```python
from build123d import *

# Parameters (mm, degrees)
F0_W      = 670
F0_H      = 678
F1_DEPTH  = 540
F2_R      = 31.5
F3_DEPTH  = 125
F4_W      = 290
F4_H      = 33
F5_DEPTH  = 670
F6_R      = 190
F7_DEPTH  = 670
F8_W      = 105.455173281
F8_H      = 190
F9_DEPTH  = 670
F11_DEPTH = 15


with BuildPart() as f1:
    # F0 (on Front) → F1 (new body)
    with BuildSketch(Plane.XZ):
        with Locations((1.9415970892, 64.8658148712)):
            Rectangle(F0_W, F0_H)
    extrude(amount=-F1_DEPTH)

    # F2 (on face) → F3 (cut)
    with BuildSketch(Plane.XY.offset(403.8658148712)):
        with Locations((1.9415970892, 457)):
            Circle(F2_R)
    extrude(amount=-F3_DEPTH, mode=Mode.SUBTRACT)

    # F4 (on face) → F5 (cut)
    with BuildSketch(Plane.YZ.offset(336.9415970892)):
        with Locations((395, 262.3658148712)):
            Rectangle(F4_W, F4_H)
    extrude(amount=-F5_DEPTH, mode=Mode.SUBTRACT)

    # F6 (on face) → F7 (cut)
    with BuildSketch(Plane.YZ.offset(336.9415970892)):
        with Locations((270, -4.1341851288)):
            Circle(F6_R)
    extrude(amount=-F7_DEPTH, mode=Mode.SUBTRACT)

    # F8 (on face) → F9 (cut)
    with BuildSketch(Plane.YZ.offset(336.9415970892)):
        with Locations((487.2724133595, -4.1341851288)):
            Rectangle(F8_W, F8_H)
    extrude(amount=-F9_DEPTH, mode=Mode.SUBTRACT)

    # F10 (on face) → F11 (cut)
    with BuildSketch(Plane.XZ):
        Polygon((-285.0584029108, 403.8658148712), (-333.0584029108, 403.8658148712), (-333.0584029108, 355.8658148712), (-45.7536410061, 64.8658148712), (-333.0584029108, -226.1341851288), (-333.0584029108, -274.1341851288), (-285.0584029108, -274.1341851288), (1.9415970892, 16.5571331991), (288.9415970892, -274.1341851288), (336.9415970892, -274.1341851288), (336.9415970892, -226.1341851288), (49.6368351844, 64.8658148712), (336.9415970892, 355.8658148712), (336.9415970892, 403.8658148712), (288.9415970892, 403.8658148712), (1.9415970892, 113.1744965432), align=None)
    extrude(amount=-F11_DEPTH, mode=Mode.SUBTRACT)


solid = f1.part
```
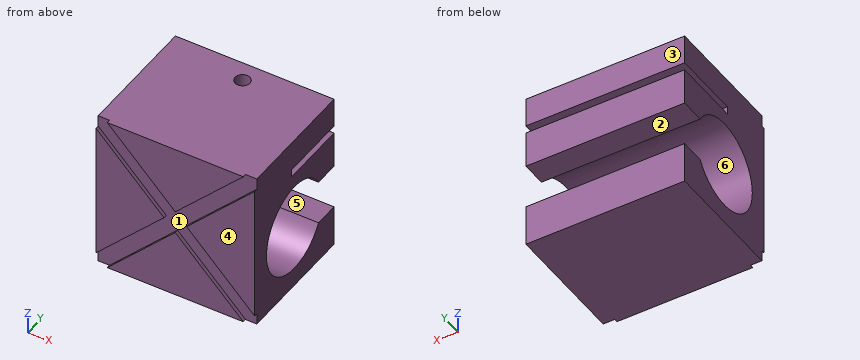
Could you check a few things on this model? Use its own coordinates, in mm. Face numbers are marked on the shaded views. A direction names the side the tool comes from. Round coordinates to 2 decimals unless told otherwise and drop trailing zeros. Order: outer loops, then holes, each group sorted by start corner. A loop starts at its lowest first (then second) coordinate and runs counter-clockwise, first axis right, second up. Notation, with made-up numbers: M -38.5,-10.5 L -20.5,-10.5 A7 cw -20.5,-1.5 Z; hole C 43,-8.5 d6. An arc over 180 degrees is marked long. One line per question, with ' | ' between items. Start each with the question number.
(1) Please list where these lines run through material, in increasing order: line 1 along Z through (x, y) = (99.5, 439); line 2 along Z through (x, y) = (-120, 270); line 3 along Y through (x, z) = (143.5, -67).
(2) Suppose I cut it at B-B on y = 123.5. List the corners of the cut face in (x, z) for me.
(3) Suppose I cut it at A-A on y = 498. List the corners of the cut face in (x, z) for me, then the cut area to 3 significant figures.
(4) Suppose I cut it at C-C on x = -20. List the corners of the cut face in (y, z) for me, then the cut area to 3 significant figures.
(5) Suppose I cut it at D-D on z = 316. List the corners of the cut face in (x, y) for me.
(6) For the marked faces 1, 2 and 3, which set-ups out of +Z, -Z, +X, -X, +Y, -Y let a thin tool reach every point of the face, with its end or its side?
(7) For P1, Ø2, axis at x = 55, z = 38, coming from the -Y side; P2, Ø16.5, axis at x = -14.5, z = 258.5, coming from the +Y side, each with a flat end and sliding along its axis, tell me the tip position at first contact or that it passes through.
(8) Thinking about a two-plate mould opening in Y: for the marked faces 4, 5 and 6, which applies, +Y half, -Y half, draft (parallel to the pull), parting line (faces both ways), or undercut?
Geometry results:
1) line 1: -274.13 to -99.13, 90.87 to 245.87, 278.87 to 403.87 | line 2: -274.13 to -194.13, 185.87 to 245.87, 278.87 to 403.87 | line 3: 15 to 90.7
2) outline: M -333.06,-274.13 L 336.94,-274.13 L 336.94,-125.12 L -333.06,-125.12 Z; M -333.06,116.85 L 336.94,116.85 L 336.94,403.87 L -333.06,403.87 Z
3) outline: M -333.06,-274.13 L 336.94,-274.13 L 336.94,-99.13 L -333.06,-99.13 Z; M -333.06,90.87 L 336.94,90.87 L 336.94,245.87 L -333.06,245.87 Z; M -333.06,278.87 L 336.94,278.87 L 336.94,403.87 L -333.06,403.87 Z | area: 305,000 mm²
4) outline: M 0,-274.13 L 540,-274.13 L 540,-99.13 L 434.54,-99.13 A190 cw long 434.54,90.87 L 540,90.87 L 540,245.87 L 250,245.87 L 250,278.87 L 434.4,278.87 L 434.4,403.87 L 0,403.87 L 0,135.4 L 15,135.4 L 15,-5.67 L 0,-5.67 Z; M 479.6,278.87 L 540,278.87 L 540,403.87 L 479.6,403.87 Z | area: 219,000 mm²
5) outline: M -333.06,0 L -293.7,0 L -293.7,15 L -198.31,15 L -198.31,0 L 202.19,0 L 202.19,15 L 297.58,15 L 297.58,0 L 336.94,0 L 336.94,540 L -333.06,540 Z; hole C 1.94,457 d63
6) face 1: -Y | face 2: +X, -X, +Y | face 3: +Z, -Z, +X, -X, +Y
7) P1: y = 15 | P2: y = 250
8) face 4: -Y half | face 5: draft | face 6: undercut
